Input: dimensioned drawing with shaded views. Units: mm. Origin: part minimum x, y, z. A direction names the side the tool comes from. Coordinates: 2 decimals unless noted, no trailing zeros. Write each loop counter-clockwise with the first axis right and the second up, starting at its lowest first coordinate (ties: lowest second). Pieces come first, ordered by that corner, then holes. Notation, with made-up numbers: (-39, 44.5) -> (10, 44.5) arc R20 ccw to (10, 67.5) -> close; hole circle Ø10 at (28, 43.5). An arc over 180 degrees is marked (long way). One line per item, written item: value. Start each with the question number.
1. Section query A-A, the plane x = 17.5. Output: boundary loops of the cut face in (y, z).
2. Mould query, pull axis Y, two halves, no side actions, for the marked faces 1, 2 and 3. Classes: released by +Y, released by -Y, zero draft, split by the parting line, or undercut.
3. Section query C-C, the plane z = 33. Output: boundary loops of the cut face in (x, y).
4. Access query for the marked faces 4 and 5. Directions: +Z, -Z, +X, -X, +Y, -Y. A direction counts if a zero-diameter tool reaches every point of the face in a straight line with its end or side. Return the directions, or none.
5. Line query: line 1 (Y direction, x = 54, z = 32); line 2 (X direction, y = 4.75, z = 14.5) (1 decimal); line 3 (Z direction, x = 16, y = 2). Output: solid intervals per line, ascending.
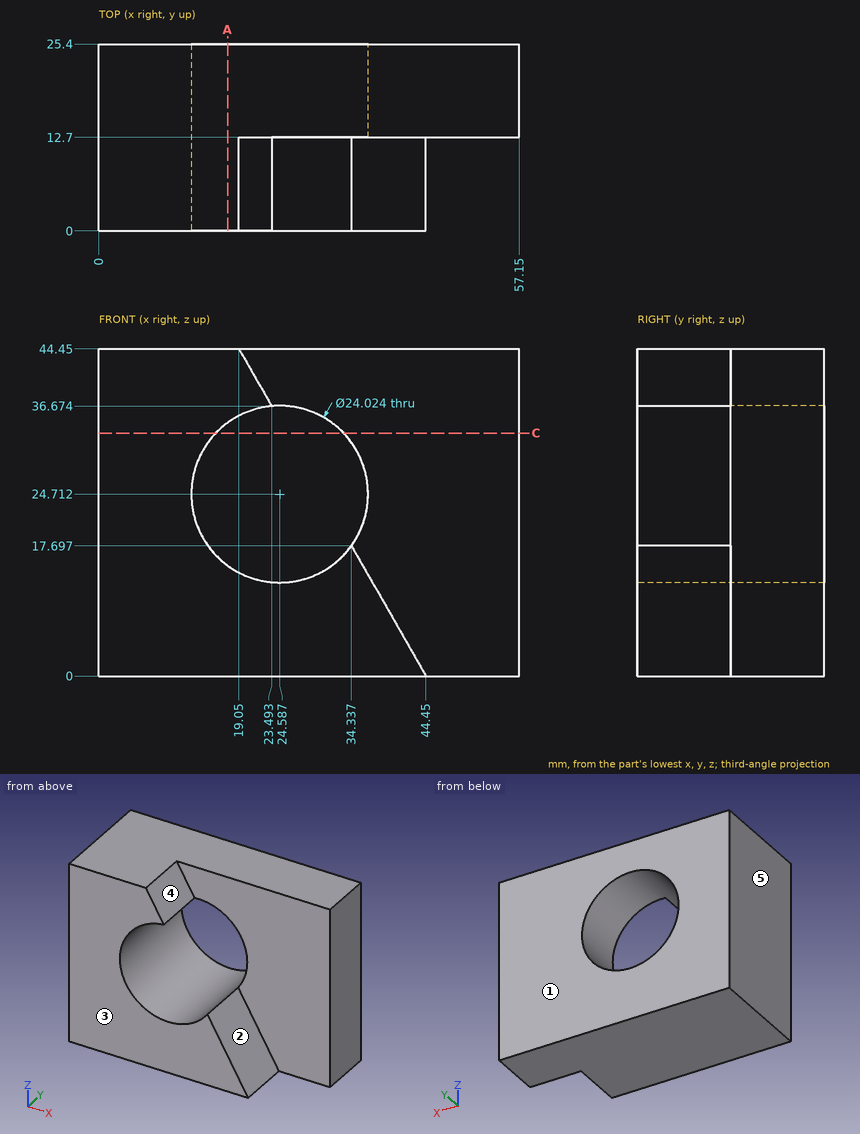
Computed values:
1. outline: (0, 0) -> (25.4, 0) -> (25.4, 15.01) -> (0, 15.01) -> close; (0, 34.41) -> (25.4, 34.41) -> (25.4, 44.45) -> (0, 44.45) -> close
2. face 1: released by +Y
2. face 2: zero draft
2. face 3: released by -Y
3. outline: (0, 0) -> (15.89, 0) -> (15.89, 25.4) -> (0, 25.4) -> close; (33.28, 12.7) -> (57.15, 12.7) -> (57.15, 25.4) -> (33.28, 25.4) -> close
4. face 4: +Z, +X, -Y
4. face 5: +Z, -Z, -X, +Y, -Y
5. line 1: y = 12.7 to 25.4
5. line 2: x = 0 to 18.3, 30.9 to 36.2
5. line 3: z = 0 to 16.31, 33.11 to 44.45
